For this review, take the finished solid that the model builds, in its own axes (mm). Give positions to 0.01 mm unless a question says otherwise; leave off trailing zeros. Order: outer loops, then holes, each group sorted by start corner. A loop starts at its lowest first (then second) coordinate and runs counter-clockwise, first axis right, second up. Notation, with made-up numbers: M -7,50 L 20,50 A12 ccw 20,55 Z; hole C 24.5,66 d3. An arc over 180 degrees is marked long. Answer as CSV lines item,"result". Start each with the question number.
1. We need section B-B, the plane z = 30.5. Give the boundary of the cut face in (x, y), and give its area (3 significant figures).
2. We need section A-A, the plane x = 15.5. Give the boundary of the cut face in (y, z), and give its area (3 significant figures).
3. For line 1 along X through (y, z) = (1, 122.5); line 2 along Z through (x, y) = (31, -3.75); line 3 along Y through (x, z) = (-5.1, 162.5), list the stretches that pass through material, from the lowest coordinate up.
4. Clearance check with flat-ended pins moving along their axes: P1, Ø1.8, axis at y = -3.45, z = -2.21, coming from the +X side; P2, Ø2.5, axis at y = -3.45, z = -2.21, coming from the -X side. State where each tip first meets the part, or that it passes through.
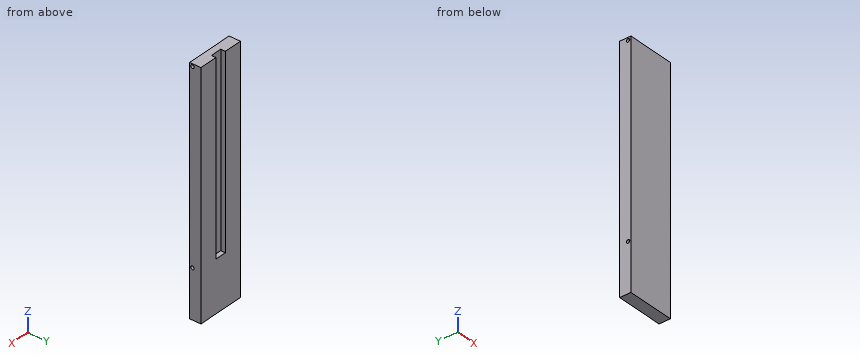
Autodesk Inventor part; units mm, degrees
ref_plane "YZ Plane" through (0, 0, 0) normal (1, 0, 0) x (0, 1, 0)
ref_plane "XZ Plane" through (0, 0, 0) normal (0, 1, 0) x (-1, 0, 0)
ref_plane "XY Plane" through (0, 0, 0) normal (0, 0, 1) x (1, 0, 0)
sketch "Sketch1" plane through (0, 0, 0) normal (0, 0, 1) x (1, 0, 0)
  line L0 (-7.378, 4.0507) -> (34.622, 4.0507)
  line L1 (34.622, 4.0507) -> (34.622, -5.9493)
  line L2 (34.622, -5.9493) -> (-7.378, -5.9493)
  line L3 (-7.378, -5.9493) -> (-7.378, 4.0507)
  line L4 (8.622, 4.0507) -> (8.622, 0.0507)
  line L5 (18.622, 4.0507) -> (18.622, 0.0507)
  line L6 (18.622, 0.0507) -> (8.622, 0.0507)
  point P0 (0, 0)
extrude "Extrusion1" add sketch "Sketch1" against normal blind 45
extrude "Extrusion2" add sketch "Sketch1" along normal blind 165 contours L0 L4 L6 L5 L1 L2 L3
sketch "Sketch2" plane through (34.622, -5.9493, -45) normal (1, 0, 0) x (0, 0, -1)
  line L0 (0, 0) -> (0, 10)
  line L1 (0, 0) -> (-210, 0)
  line L2 (-210, 10) -> (0, 10)
  circle A0 centre (-42.793, 2.5) radius 1.5
  point P0 (-45, 5.9493)
hole "Hole1" at (34.622, -3.4493, -2.207) direction (-1, 0, 0) diameter 3 depth 5 tip angle 118
sketch "Sketch3" plane through (34.622, -5.9493, -45) normal (1, 0, 0) x (0, 0, -1)
  line L0 (0, 0) -> (-210, 0)
  line L1 (-210, 0) -> (-207.5, 0)
  line L2 (-207.5, 0) -> (-207.5, 2.5)
  circle A0 centre (-207.5, 2.5) radius 1.5
  point P0 (-45, 5.9493)
  dimension "d19" = 2.5
  dimension "d20" = 2.5
  dimension "d21" = 3
hole "Hole2" at (34.622, -3.4493, 162.5) direction (-1, 0, 0) diameter 3 depth 5 tip angle 118
sketch "Sketch4" plane through (-7.378, -5.9493, -45) normal (-1, 0, 0) x (0, 0, 1)
  circle A0 centre (207.5, 2.5) radius 1.5
  circle A1 centre (207.5, 2.5) radius 1.5
  circle A2 centre (42.793, 2.5) radius 1.5
  circle A3 centre (42.793, 2.5) radius 1.5
  point P0 (45, 5.9493)
hole "Hole3" at (-7.378, -3.4493, 162.5) direction (1, 0, 0) diameter 3 depth 5 tip angle 118
hole "Hole4" at (-7.378, -3.4493, -2.207) direction (1, 0, 0) diameter 3 depth 5 tip angle 118
thread "Thread1"
thread "Thread2"
thread "Thread3"
thread "Thread4"
properties part number "sina" material "Lead"
Result set:
1,outline,"M -7.38,-5.95 L 34.62,-5.95 L 34.62,4.05 L 18.62,4.05 L 18.62,0.05 L 8.62,0.05 L 8.62,4.05 L -7.38,4.05 Z"
1,area,"380 mm2"
2,outline,"M -5.95,-45 L 4.05,-45 L 4.05,0 L 0.05,0 L 0.05,165 L -5.95,165 Z"
2,area,"1,440 mm2"
3,line 1,"-7.38 to 8.62, 18.62 to 34.62"
3,line 2,"-45 to -3.68, -0.74 to 161.03, 163.97 to 165"
3,line 3,"-5.95 to -4.95, -1.95 to 4.05"
4,P1,"x = 29.26"
4,P2,"x = -2.23"
